The model under review builds one solid part; all positions refer to its coordinate system, in mm. Face numbers are marked on the shaded views. A direction names the side the tool comes from. Round coordinates to 2 decimals unless told otherwise and drop trailing zeros. Order: outer loops, then holes, each group sorted by start corner. A loop starts at its lowest first (then second) coordinate and runs counter-clockwise, first axis right, second up.
1) Consider section D-D (x = 24). Give the boundary of the cut face in (y, z).
2) Consider section C-C (y = -45.5). Give the boundary of the cut face in (x, z).
3) Mouldability with a two-part tool opening along Y and no side actions: class the marked faces 1, 2, 3 and 4 as pulls with the +Y half, pulls with the -Y half, needs draft (parallel to the pull), parting line crosses it, or undercut.
4) Machinability: for the marked faces 5, 6, 7, 8 and 9, which of the approach directions +Z, -Z, +X, -X, +Y, -Y give a long, thin tool a straight path to every point of the face, cutting with its end or side? Answer none if there is none.
5) To check wall thickness, follow L1, parallel to Z at x = -0.4, y = 45.5; L2, parallel to X at y = 25.5, z = -0.25; L3, parallel to Z at x = 36, y = -8. State the ranges of each line that lie inside material, in increasing order.
6) Consider section B-B (x = 33). Give the boundary of the cut face in (y, z).
7) Consider section A-A (z = 0). Give the number of separate pieces and of enclosed holes in the cut face, then the cut area to 3 significant figures.
8) Clearance check with flat-ended pins moving along their axes: P1, Ø4, axis at x = 20.5, y = -26, coming from the -Z side; P2, Ø7.5, axis at x = 39.5, y = 7.5, coming from the +Z side; P3, Ø3.5, axis at x = 25, z = -2.5, coming from the -Y side; P4, Ø4, axis at x = 19, z = 10, coming from the +Y side (3 decimals). State where each tip first meets the part, or that it passes through.
from build123d import *

# Parameters (mm, degrees)
EXTRUDE_1_DEPTH     = 6.5
SKETCH_2_W          = 28
SKETCH_2_H          = 100
SKETCH_2_R          = 2.5
EXTRUDE_2_DEPTH     = 0.75
SKETCH_3_W          = 6
SKETCH_3_H          = 31
CUT_EXTRUDE_1_DEPTH = 5
SKETCH_4_W          = 13.5
SKETCH_4_H          = 5.5
CUT_EXTRUDE_2_DEPTH = 5
EXTRUDE_3_DEPTH     = 2.75
FILLET_1_R          = 1
FILLET_2_R          = 1


with BuildPart() as part:
    # 草图1 → 凸台-拉伸1 (new, symmetric)
    with BuildSketch(Plane.XY):
        Polygon((0, 1.01114255), (0, 0), (35, 0), (35, 27.496864511), (6, 27.496864511), (6, 37.5), (0, 37.5), align=None)
        Polygon((35, 0), (0, 0), (0, -1.01114255), (0, -37.5), (6, -37.5), (6, -27.496864511), (35, -27.496864511), align=None)
    extrude(amount=EXTRUDE_1_DEPTH, both=True)

    # 草图2 → 凸台-拉伸2 (add, symmetric)
    with BuildSketch(Plane.ZY):
        Rectangle(SKETCH_2_W, SKETCH_2_H)
        with Locations(Location((0, -45.5, 0), (0, 0, 270))):
            Circle(SKETCH_2_R, mode=Mode.SUBTRACT)
        with Locations(Location((0, 45.5, 0), (0, 0, 90))):
            Circle(SKETCH_2_R, mode=Mode.SUBTRACT)
    extrude(amount=EXTRUDE_2_DEPTH, both=True)

    # 草图3 → 切除-拉伸1 (cut)
    with BuildSketch(Plane(origin=(35, 0, 0), x_dir=(0, 0, -1), z_dir=(1, 0, 0))):
        Rectangle(SKETCH_3_W, SKETCH_3_H)
    extrude(amount=-CUT_EXTRUDE_1_DEPTH, mode=Mode.SUBTRACT)

    # 草图4 → 切除-拉伸2 (cut)
    with BuildSketch(Plane.XZ.offset(27.496864511)):
        with Locations((21.75, 0)):
            Rectangle(SKETCH_4_W, SKETCH_4_H)
    extrude(amount=-CUT_EXTRUDE_2_DEPTH, mode=Mode.SUBTRACT)

    # 草图5 → 凸台-拉伸3 (add, symmetric)
    with BuildSketch(Plane.XY):
        with BuildLine():
            Line((30, -15.5), (30, 15.5))
            Line((30, 15.5), (35, 15.5))
            ThreePointArc((35, 15.5), (42.36590029, 12.263395074), (44.963698746, 4.648702584))
            Line((44.963698746, 4.648702584), (43.892853324, -7.884615385))
            ThreePointArc((43.892853324, -7.884615385), (40.85399272, -13.335990728), (35, -15.5))
            Line((35, -15.5), (30, -15.5))
        make_face()
    extrude(amount=EXTRUDE_3_DEPTH, both=True)

    # 圆角1
    fillet_1_edges = [part.edges().sort_by_distance(p)[0] for p in [
        (3.375, -37.5, 6.5),
        (3.375, -37.5, -6.5),
        (3.375, 37.5, 6.5),
        (3.375, 37.5, -6.5),
    ]]
    fillet(fillet_1_edges, radius=FILLET_1_R)

    # 圆角2
    fillet_2_edges = [part.edges().sort_by_distance(p)[0] for p in [
        (20.5, 27.496864511, -6.5),
        (35, 0, -6.5),
        (20.5, -27.496864511, -6.5),
        (35, 27.496864511, 0),
        (35, -27.496864511, 0),
        (20.5, -27.496864511, 6.5),
        (35, 0, 6.5),
        (20.5, 27.496864511, 6.5),
    ]]
    fillet(fillet_2_edges, radius=FILLET_2_R)


solid = part.part
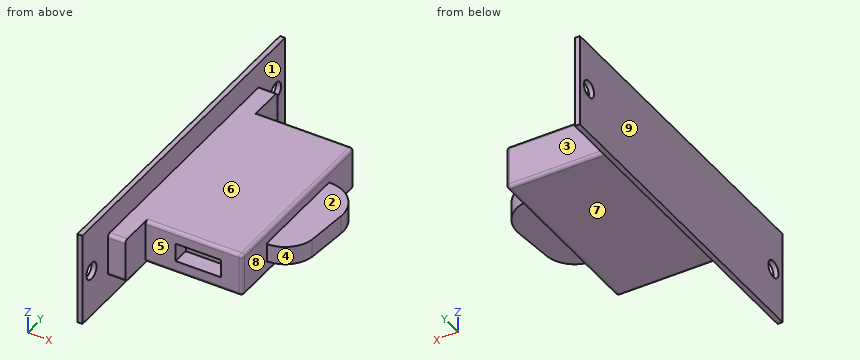
Answer below:
1. outline: (-27.5, -5.5) arc R1 ccw to (-26.5, -6.5) - (26.5, -6.5) arc R1 ccw to (27.5, -5.5) - (27.5, 5.5) arc R1 ccw to (26.5, 6.5) - (-26.5, 6.5) arc R1 ccw to (-27.5, 5.5) - (-27.5, 2.75) - (-22.5, 2.75) - (-22.5, -2.75) - (-27.5, -2.75) - close
2. outline: (-0.75, -14) - (0.75, -14) - (0.75, -2.5) - (-0.75, -2.5) - close; (-0.75, 2.5) - (0.75, 2.5) - (0.75, 14) - (-0.75, 14) - close
3. face 1: needs draft
3. face 2: undercut
3. face 3: pulls with the +Y half
3. face 4: pulls with the -Y half
4. face 5: +Z, -Z, +X, -Y
4. face 6: +Z, +X, +Y, -Y
4. face 7: -Z, +X, +Y, -Y
4. face 8: +X
4. face 9: +Z, -Z, -X, +Y, -Y
5. L1: z = -14 to -2.5, 2.5 to 14
5. L2: x = -0.75 to 35
5. L3: z = -2.75 to 2.75
6. outline: (-27.5, -5.5) arc R1 ccw to (-26.5, -6.5) - (26.5, -6.5) arc R1 ccw to (27.5, -5.5) - (27.5, 5.5) arc R1 ccw to (26.5, 6.5) - (-26.5, 6.5) arc R1 ccw to (-27.5, 5.5) - close; hole (-15.5, -3) - (15.5, -3) - (15.5, -2.75) - (-15.5, -2.75) - close; hole (-15.5, 2.75) - (15.5, 2.75) - (15.5, 3) - (-15.5, 3) - close
7. separate pieces: 3
7. enclosed holes: 0
7. area: 2,310 mm2
8. P1: stops at z = -6.5
8. P2: stops at z = 2.75
8. P3: stops at y = -27.5
8. P4: passes through
